from build123d import *

# Parameters (mm, degrees)
SKETCH_1_W      = 113
SKETCH_1_H      = 72
EXTRUDE_1_DEPTH = 19
SKETCH_2_W      = 7.344019186
SKETCH_2_H      = 17.001907431
EXTRUDE_2_DEPTH = 5
SKETCH_3_R      = 2.471853224
SKETCH_3_R_2    = 2.395721662
EXTRUDE_3_DEPTH = 10


with BuildPart() as part:
    # 草图1 → 凸台-拉伸1 (new body)
    with BuildSketch(Plane(origin=(0, 0, 0), x_dir=(1, 0, 0), z_dir=(0, 1, 0))):
        with Locations((56.5, -36)):
            Rectangle(SKETCH_1_W, SKETCH_1_H)
    extrude(amount=EXTRUDE_1_DEPTH)

    # 草图2 → 凸台-拉伸2 (add)
    with BuildSketch(Plane(origin=(113, 0, 0), x_dir=(0, 0, -1), z_dir=(1, 0, 0))):
        with Locations((-5.329755024, 10.281536394)):
            Rectangle(SKETCH_2_W, SKETCH_2_H)
    extrude(amount=EXTRUDE_2_DEPTH)

    # 草图3 → 凸台-拉伸3 (add)
    with BuildSketch(Plane(origin=(118, 0, 0), x_dir=(0, 0, -1), z_dir=(1, 0, 0))):
        with Locations((-5.672341685, 14.927563873)):
            Circle(SKETCH_3_R)
        with Locations((-5.672341685, 6.978123812)):
            Circle(SKETCH_3_R_2)
    extrude(amount=EXTRUDE_3_DEPTH)


solid = part.part
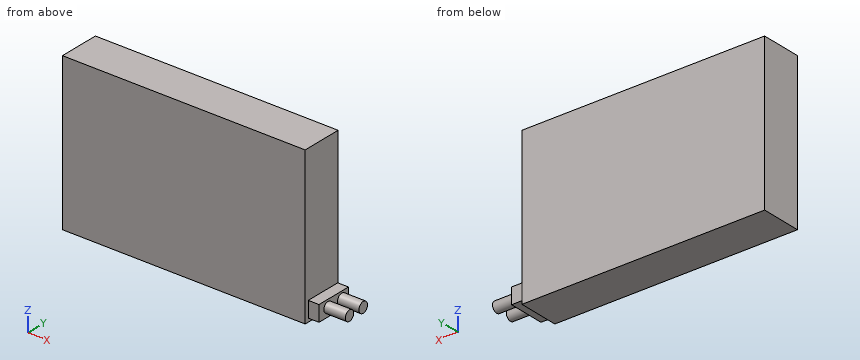
Design review of the part built by this model. Coordinates are the model's own, in mm. Give positions to 0.01 mm unless a question says otherwise; leave off trailing zeros. Order: outer loops, then holes, each group sorted by start corner. A loop starts at its lowest first (then second) coordinate and runs counter-clockwise, first axis right, second up.
1. Add section A-A, the plane y = 11. State the section outline as (x, z) points, then the cut area to 3 significant figures.
Solution:
outline: (0, 0) - (113, 0) - (113, 1.66) - (118, 1.66) - (118, 9) - (113, 9) - (113, 72) - (0, 72) - close
area: 8,170 mm2
2. For pin 1 Ø3.5 at (y, z) = (10, 6.5) entering from +X; pin 2 Ø8 at (y, z) = (16, 48) entering from +X; pin 3 Ø1.5 at (x, z) = (114.5, 4.5) entering from +Y; pin 4 Ø2.5 at (x, y) = (116.5, 8.5) entering from -Z, all flat-tipped, find the tip position at first contact; note any pin that passes through.
Solution:
pin 1: stops at x = 128
pin 2: stops at x = 113
pin 3: stops at y = 18.78
pin 4: stops at z = 1.66
3. Add section D-D, the plane z = 20.5. State the section outline as (x, y) points, then the cut area to 3 significant figures.
Solution:
outline: (0, 0) - (113, 0) - (113, 19) - (0, 19) - close
area: 2,150 mm2
4. Add section B-B, the plane z = 5. State the section outline as (x, y) points, then the cut area to 3 significant figures.
Solution:
outline: (0, 0) - (113, 0) - (113, 1.78) - (118, 1.78) - (118, 4.68) - (128, 4.68) - (128, 9.28) - (118, 9.28) - (118, 12.55) - (128, 12.55) - (128, 17.31) - (118, 17.31) - (118, 18.78) - (113, 18.78) - (113, 19) - (0, 19) - close
area: 2,330 mm2
5. Add section C-C, the plane x = 119.5. State the section outline as (y, z) points.
Solution:
outline: circle Ø4.79 at (6.98, 5.67); circle Ø4.94 at (14.93, 5.67)
6. To check wall thickness, follow L1, parallel to X at y = 5, z = 40; L2, parallel to X at y = 3, z = 8.5; L3, parallel to Z at x = 121.5, y = 16. State the ranges of each line that lie inside material, in increasing order.
Solution:
L1: x = 0 to 113
L2: x = 0 to 118
L3: z = 3.45 to 7.9
